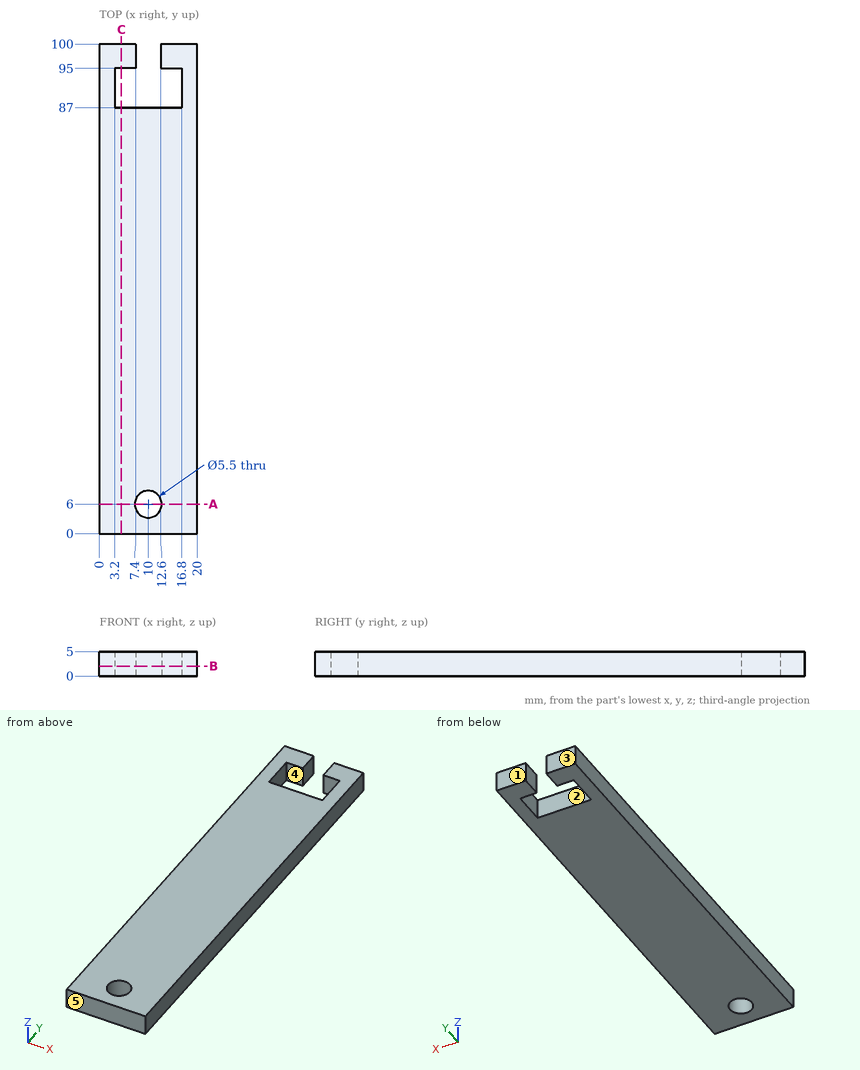
Answer from the drawing. Dimensions are ordinates in mm from the lowest x, y and z of the part. A direction names the side the tool comes from. Coordinates: 2 decimals unless noted, no trailing zeros. Loops run counter-clockwise (first coordinate to the right, second up) from the corner with the lowest first, then second, coordinate; pieces in that order, holes last. Notation, with made-up numbers: (75, 34) -> (105, 34) arc R21 cw to (105, 61) -> close; hole circle Ø6 at (59.5, 65). An arc over 180 degrees is marked (long way). Answer as CSV lines item,"result".
Q1. Each of these flat-tipped pins is pushed along its axis until it touches: pin 1 (2 mm diameter, centred on x = 11.5, z = 1.5, fed in from +Y); pin 2 (6 mm diameter, centred on x = 2.5, y = 67, fed in from -Z). Where does it stop, or does it pass through?
Findings:
pin 1,"stops at y = 87"
pin 2,"stops at z = 0"
Q2. For a pull along Y with two mould halves and no side action, classify the marked faces 3, 4 and 5 as +Y half, -Y half, draft (parallel to the pull), parting line (faces both ways), or undercut.
Findings:
face 3,"+Y half"
face 4,"undercut"
face 5,"-Y half"
Q3. The part is cut by section B-B on z = 2. Write down the section's boundary in (x, y), and give its area (3 significant figures).
Findings:
outline,"(0, 0) -> (20, 0) -> (20, 100) -> (12.6, 100) -> (12.6, 95) -> (16.8, 95) -> (16.8, 87) -> (3.2, 87) -> (3.2, 95) -> (7.4, 95) -> (7.4, 100) -> (0, 100) -> close; hole circle Ø5.5 at (10, 6)"
area,"1,840 mm²"
Q4. The part is cut by section A-A on y = 6. Write down the section's boundary in (x, z), and give its area (3 significant figures).
Findings:
outline,"(0, 0) -> (7.25, 0) -> (7.25, 5) -> (0, 5) -> close; (12.75, 0) -> (20, 0) -> (20, 5) -> (12.75, 5) -> close"
area,"72.5 mm²"
Q5. Find the intervals of material crossed by probe 1 along Y at (x, z) = (16, 1.6); probe 2 along Y at (x, z) = (10, 2.1); probe 3 along X at (y, z) = (5.5, 4.5), in increasing order.
Findings:
probe 1,"y = 0 to 87, 95 to 100"
probe 2,"y = 0 to 3.25, 8.75 to 87"
probe 3,"x = 0 to 7.3, 12.7 to 20"
Q6. The part is cut by section C-C on x = 4.5. Write down the section's boundary in (y, z).
Findings:
outline,"(0, 0) -> (87, 0) -> (87, 5) -> (0, 5) -> close; (95, 0) -> (100, 0) -> (100, 5) -> (95, 5) -> close"
Q7. A tool of negligible diameter and unlimited length cuts with its end or side. For the marked faces 1 and 2, from which of +Z, -Z, +X, -X, +Y, -Y can it reach the whole face along a straight path? Write none if from no direction.
Findings:
face 1,"+Z, -Z, +X, -X, +Y"
face 2,"+Z, -Z"
